Study the drawing (mm; zero at the part's minimum x, y, z) and answer. Give positions to 0.01 mm unless a question says otherwise; leave off trailing zeros. Write each loop counter-clockwise with the first axis right and the second up, starting at its lowest first coordinate (ties: lowest second). Pieces come first, ordered by that corner, then holes.
1) Determine the mould class of the marked faces 1, 2 and 3 for opening direction X: pulls with the +X half, pulls with the -X half, needs draft (parallel to the pull), parting line crosses it, or undercut.
2) Straight lines are drawn through the part: probe 1 along X at (y, z) = (2.15, 27.5); probe 2 along X at (y, z) = (1.2, 7.5); probe 3 along Z at (x, y) = (7, 1.95) (1 decimal). For each, find the intervals that lie inside material, in ascending order.
3) Given pin 1 Ø0.9 at (y, z) = (1, 28) entering from -X; pin 2 Ø7 at (x, z) = (7.5, 7.5) entering from +Y; pin 3 Ø5 at (x, z) = (7.5, 27.5) entering from +Y; pin 4 Ø1.5 at (y, z) = (1.5, 23) entering from -X (1 decimal), each flat-ended and moving along its own axis, determine where each tip first touches the part or whether it passes through.
4) Find section A-A (x = 7.5). Determine the outline of the cut face in (y, z).
5) Find section D-D (x = 5.25). Determine the outline of the cut face in (y, z) (1 decimal), plus the area to 3 significant figures.
6) Find section B-B (y = 1.35). Determine the outline of the cut face in (x, z), plus the area to 3 significant figures.
7) Find section C-C (z = 37.5). Determine the outline of the cut face in (x, y).
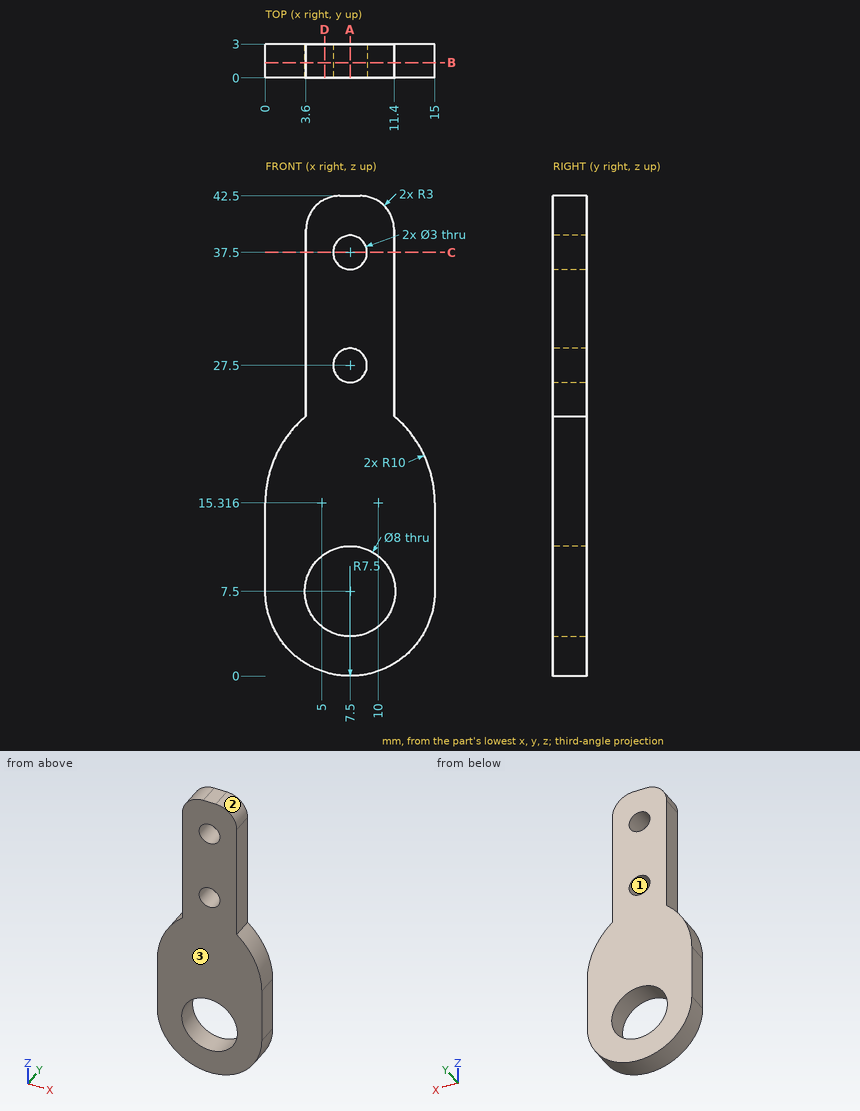
Results:
1. face 1: undercut
1. face 2: pulls with the +X half
1. face 3: needs draft
2. probe 1: x = 3.6 to 6, 9 to 11.4
2. probe 2: x = 0 to 3.5, 11.5 to 15
2. probe 3: z = 0 to 3.5, 11.5 to 26.1, 28.9 to 36.1, 38.9 to 42.5
3. pin 1: stops at x = 3.6
3. pin 2: passes through
3. pin 3: stops at y = 3
3. pin 4: stops at x = 2.8
4. outline: (0, 0) - (3, 0) - (3, 3.5) - (0, 3.5) - close; (0, 11.5) - (3, 11.5) - (3, 26) - (0, 26) - close; (0, 29) - (3, 29) - (3, 36) - (0, 36) - close; (0, 39) - (3, 39) - (3, 42.5) - (0, 42.5) - close
5. outline: (0, 0.3) - (3, 0.3) - (3, 4.2) - (0, 4.2) - close; (0, 10.8) - (3, 10.8) - (3, 42.2) - (0, 42.2) - close
5. area: 106 mm2
6. outline: (0, 7.5) arc R7.5 ccw to (15, 7.5) - (15, 15.32) arc R10 ccw to (11.4, 23) - (11.4, 39.5) arc R3 ccw to (8.4, 42.5) - (6.6, 42.5) arc R3 ccw to (3.6, 39.5) - (3.6, 23) arc R10 ccw to (0, 15.32) - close; hole circle Ø8 at (7.5, 7.5); hole circle Ø3 at (7.5, 27.5); hole circle Ø3 at (7.5, 37.5)
6. area: 388 mm2
7. outline: (3.6, 0) - (6, 0) - (6, 3) - (3.6, 3) - close; (9, 0) - (11.4, 0) - (11.4, 3) - (9, 3) - close
